Verification items for the finished model (mm, model axes). Face numbers are marked on the shaded views. A direction names the side the tool comes from. Round coordinates to 2 decimals unless told otherwise and drop trailing zeros. Write each loop counter-clockwise with the first axis right and the second up, starting at its lowest first coordinate (ties: lowest second). Pieces come first, ordered by that corner, then holes. Notation, with made-up numbers: M 3.5,49 L 55.5,49 A14 ccw 55.5,58 Z; hole C 63,26 d9. An arc over 180 degrees is marked long. One line per question, with ' | ' between items.
from build123d import *

# Parameters (mm, degrees)
F0_R     = 12.5
F0_R_2   = 18
F0_R_3   = 16
F0_R_4   = 8.5
F0_R_5   = 3.5
F1_DEPTH = 20
F2_DEPTH = 2
F3_R     = 1.5
F4_SIZE  = 1
F5_SIZE  = 1


# Not quite as in the source:
# - a feature names something its author has since deleted; it is built from what else it names


with BuildPart() as f1:
    # F0 (on Top) → F1 (new body)
    with BuildSketch(Plane.XY):
        with BuildLine():
            Line((82.5, 50), (-82.5, 50))
            ThreePointArc((-82.5, 50), (-86.0355339059, 48.5355339059), (-87.5, 45))
            Line((-87.5, 45), (-87.5, -45))
            ThreePointArc((-87.5, -45), (-86.0355339059, -48.5355339059), (-82.5, -50))
            Line((-82.5, -50), (82.5, -50))
            ThreePointArc((82.5, -50), (86.0355339059, -48.5355339059), (87.5, -45))
            Line((87.5, -45), (87.5, 45))
            ThreePointArc((87.5, 45), (86.0355339059, 48.5355339059), (82.5, 50))
        make_face()
        with Locations((-70, -34.5)):
            Circle(F0_R, mode=Mode.SUBTRACT)
        with BuildLine():
            ThreePointArc((-32.5, -34.5), (-45, -47), (-57.5, -34.5))
            ThreePointArc((-57.5, -34.5), (-45, -22), (-32.5, -34.5))
        make_face(mode=Mode.SUBTRACT)
        with BuildLine():
            ThreePointArc((-7.5, -34.5), (-20, -47), (-32.5, -34.5))
            ThreePointArc((-32.5, -34.5), (-20, -22), (-7.5, -34.5))
        make_face(mode=Mode.SUBTRACT)
        with Locations((-60, -3.5)):
            Circle(F0_R_2, mode=Mode.SUBTRACT)
        with Locations((-20, -3.5)):
            Circle(F0_R_2, mode=Mode.SUBTRACT)
        with BuildLine():
            ThreePointArc((17.5, -34.5), (5, -47), (-7.5, -34.5))
            ThreePointArc((-7.5, -34.5), (5, -22), (17.5, -34.5))
        make_face(mode=Mode.SUBTRACT)
        with BuildLine():
            ThreePointArc((20.5, -30.5), (22.5502525317, -25.5502525317), (27.5, -23.5))
            Line((27.5, -23.5), (77.5, -23.5))
            ThreePointArc((77.5, -23.5), (82.4497474683, -25.5502525317), (84.5, -30.5))
            Line((84.5, -30.5), (84.5, -38.5))
            ThreePointArc((84.5, -38.5), (82.4497474683, -43.4497474683), (77.5, -45.5))
            Line((77.5, -45.5), (27.5, -45.5))
            ThreePointArc((27.5, -45.5), (22.5502525317, -43.4497474683), (20.5, -38.5))
            Line((20.5, -38.5), (20.5, -30.5))
        make_face(mode=Mode.SUBTRACT)
        with Locations((20, -3.5)):
            Circle(F0_R_2, mode=Mode.SUBTRACT)
        with Locations((60, -3.5)):
            Circle(F0_R_2, mode=Mode.SUBTRACT)
        with BuildLine():
            ThreePointArc((82, 23), (79.9497474683, 18.0502525317), (75, 16))
            Line((75, 16), (-75, 16))
            ThreePointArc((-75, 16), (-79.9497474683, 18.0502525317), (-82, 23))
            Line((-82, 23), (-82, 40))
            ThreePointArc((-82, 40), (-79.9497474683, 44.9497474683), (-75, 47))
            Line((-75, 47), (75, 47))
            ThreePointArc((75, 47), (79.9497474683, 44.9497474683), (82, 40))
            Line((82, 40), (82, 23))
        make_face(mode=Mode.SUBTRACT)
        with BuildLine():
            Line((-75, 16), (75, 16))
            ThreePointArc((75, 16), (79.9497474683, 18.0502525317), (82, 23))
            Line((82, 23), (82, 40))
            ThreePointArc((82, 40), (79.9497474683, 44.9497474683), (75, 47))
            Line((75, 47), (-75, 47))
            ThreePointArc((-75, 47), (-79.9497474683, 44.9497474683), (-82, 40))
            Line((-82, 40), (-82, 23))
            ThreePointArc((-82, 23), (-79.9497474683, 18.0502525317), (-75, 16))
        make_face()
        with BuildLine():
            ThreePointArc((80, 23), (78.5355339059, 19.4644660941), (75, 18))
            Line((75, 18), (-75, 18))
            ThreePointArc((-75, 18), (-78.5355339059, 19.4644660941), (-80, 23))
            Line((-80, 23), (-80, 40))
            ThreePointArc((-80, 40), (-78.5355339059, 43.5355339059), (-75, 45))
            Line((-75, 45), (75, 45))
            ThreePointArc((75, 45), (78.5355339059, 43.5355339059), (80, 40))
            Line((80, 40), (80, 23))
        make_face(mode=Mode.SUBTRACT)
        with Locations((60, -3.5)):
            Circle(F0_R_2)
        with Locations((60, -3.5)):
            Circle(F0_R_3, mode=Mode.SUBTRACT)
        with Locations((20, -3.5)):
            Circle(F0_R_2)
        with Locations((20, -3.5)):
            Circle(F0_R_3, mode=Mode.SUBTRACT)
        with Locations((-20, -3.5)):
            Circle(F0_R_2)
        with Locations((-20, -3.5)):
            Circle(F0_R_3, mode=Mode.SUBTRACT)
        with Locations((-60, -3.5)):
            Circle(F0_R_2)
        with Locations((-60, -3.5)):
            Circle(F0_R_3, mode=Mode.SUBTRACT)
        with Locations((-70, -34.5)):
            Circle(F0_R)
        with Locations((-70, -34.5)):
            Circle(F0_R_4, mode=Mode.SUBTRACT)
        with Locations((-70, -34.5)):
            Circle(F0_R_4)
        with Locations((-70, -34.5)):
            Circle(F0_R_5, mode=Mode.SUBTRACT)
        with BuildLine():
            ThreePointArc((-32.5, -34.5), (-45, -22), (-57.5, -34.5))
            ThreePointArc((-57.5, -34.5), (-45, -47), (-32.5, -34.5))
        make_face()
        with Locations((-45, -34.5)):
            Circle(F0_R_4, mode=Mode.SUBTRACT)
        with Locations((-45, -34.5)):
            Circle(F0_R_4)
        with Locations((-45, -34.5)):
            Circle(F0_R_5, mode=Mode.SUBTRACT)
        with BuildLine():
            ThreePointArc((-7.5, -34.5), (-20, -22), (-32.5, -34.5))
            ThreePointArc((-32.5, -34.5), (-20, -47), (-7.5, -34.5))
        make_face()
        with Locations((-20, -34.5)):
            Circle(F0_R_4, mode=Mode.SUBTRACT)
        with Locations((-20, -34.5)):
            Circle(F0_R_4)
        with Locations((-20, -34.5)):
            Circle(F0_R_5, mode=Mode.SUBTRACT)
        with BuildLine():
            ThreePointArc((17.5, -34.5), (5, -22), (-7.5, -34.5))
            ThreePointArc((-7.5, -34.5), (5, -47), (17.5, -34.5))
        make_face()
        with Locations((5, -34.5)):
            Circle(F0_R_4, mode=Mode.SUBTRACT)
        with Locations((5, -34.5)):
            Circle(F0_R_4)
        with Locations((5, -34.5)):
            Circle(F0_R_5, mode=Mode.SUBTRACT)
        with BuildLine():
            Line((77.5, -23.5), (27.5, -23.5))
            ThreePointArc((27.5, -23.5), (22.5502525317, -25.5502525317), (20.5, -30.5))
            Line((20.5, -30.5), (20.5, -38.5))
            ThreePointArc((20.5, -38.5), (22.5502525317, -43.4497474683), (27.5, -45.5))
            Line((27.5, -45.5), (77.5, -45.5))
            ThreePointArc((77.5, -45.5), (82.4497474683, -43.4497474683), (84.5, -38.5))
            Line((84.5, -38.5), (84.5, -30.5))
            ThreePointArc((84.5, -30.5), (82.4497474683, -25.5502525317), (77.5, -23.5))
        make_face()
        with BuildLine():
            Line((27.5, -25.5), (77.5, -25.5))
            ThreePointArc((77.5, -25.5), (81.0355339059, -26.9644660941), (82.5, -30.5))
            Line((82.5, -30.5), (82.5, -38.5))
            ThreePointArc((82.5, -38.5), (81.0355339059, -42.0355339059), (77.5, -43.5))
            Line((77.5, -43.5), (27.5, -43.5))
            ThreePointArc((27.5, -43.5), (23.9644660941, -42.0355339059), (22.5, -38.5))
            Line((22.5, -38.5), (22.5, -30.5))
            ThreePointArc((22.5, -30.5), (23.9644660941, -26.9644660941), (27.5, -25.5))
        make_face(mode=Mode.SUBTRACT)
    extrude(amount=F1_DEPTH)

    # F0 (on Top) → F2 (join)
    with BuildSketch(Plane.XY):
        with Locations((-60, -3.5)):
            Circle(F0_R_3)
        with Locations((-20, -3.5)):
            Circle(F0_R_3)
        with Locations((60, -3.5)):
            Circle(F0_R_3)
        with BuildLine():
            Line((-75, 18), (75, 18))
            ThreePointArc((75, 18), (78.5355339059, 19.4644660941), (80, 23))
            Line((80, 23), (80, 40))
            ThreePointArc((80, 40), (78.5355339059, 43.5355339059), (75, 45))
            Line((75, 45), (-75, 45))
            ThreePointArc((-75, 45), (-78.5355339059, 43.5355339059), (-80, 40))
            Line((-80, 40), (-80, 23))
            ThreePointArc((-80, 23), (-78.5355339059, 19.4644660941), (-75, 18))
        make_face()
        with BuildLine():
            ThreePointArc((82.5, -30.5), (81.0355339059, -26.9644660941), (77.5, -25.5))
            Line((77.5, -25.5), (27.5, -25.5))
            ThreePointArc((27.5, -25.5), (23.9644660941, -26.9644660941), (22.5, -30.5))
            Line((22.5, -30.5), (22.5, -38.5))
            ThreePointArc((22.5, -38.5), (23.9644660941, -42.0355339059), (27.5, -43.5))
            Line((27.5, -43.5), (77.5, -43.5))
            ThreePointArc((77.5, -43.5), (81.0355339059, -42.0355339059), (82.5, -38.5))
            Line((82.5, -38.5), (82.5, -30.5))
        make_face()
        with Locations((20, -3.5)):
            Circle(F0_R_3)
    extrude(amount=F2_DEPTH)

    # F3
    f3_edges = [f1.edges().sort_by_distance(p)[0] for p in [
        (0, -50, 20),
    ]]
    fillet(f3_edges, radius=F3_R)

    # F4
    f4_edges = [f1.edges().sort_by_distance(p)[0] for p in [
        (-76, -3.5, 20),
        (-36, -3.5, 20),
        (44, -3.5, 20),
        (-78.535534, 43.535534, 20),
        (-80, 31.5, 20),
        (22.5, -30.5, 11),
        (23.964466, -26.964466, 20),
        (4, -3.5, 20),
    ]]
    chamfer(f4_edges, length=F4_SIZE)

    # F5
    f5_edges = [f1.edges().sort_by_distance(p)[0] for p in [
        (-73.5, -34.5, 20),
        (-48.5, -34.5, 20),
        (-23.5, -34.5, 20),
        (1.5, -34.5, 20),
    ]]
    chamfer(f5_edges, length=F5_SIZE)


solid = f1.part
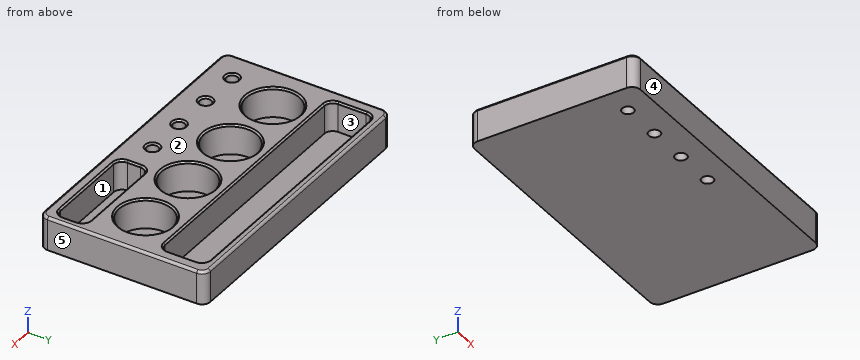
1. Tool access check on the marked faces 1 and 2. Record the directions out of +Z, -Z, +X, -X, +Y, -Y that give a thin tool (end or side, any length) a straight path to the whole face; none if there is none.
Results:
face 1: +Z | face 2: +Z, +X, -X, +Y, -Y
2. Section check D-D, the plane y = -34.5. Count the separate pieces of the cut face and the enclosed holes in it, then the cut area to 3 significant figures.
Results:
separate pieces: 5 | enclosed holes: 0 | area: 1,850 mm2
3. Section check A-A, the plane x = -20. Record the cut outline in (y, z).
Results:
outline: M -50,0 L -38,0 L -38,19 L -39,20 L -48.5,20 A1.5 ccw -50,18.5 Z; M -31,0 L 50,0 L 50,18.5 A1.5 ccw 48.5,20 L 46,20 L 45,19 L 45,2 L 18,2 L 18,19 L 17,20 L 13.5,20 L 12.5,19 L 12.5,2 L -19.5,2 L -19.5,19 L -20.5,20 L -30,20 L -31,19 Z
4. Section check C-C, the plane y = 34. Record the cut outline in (x, z).
Results:
outline: M -87.5,0 L 87.5,0 L 87.5,18.5 A1.5 ccw 86,20 L 81,20 L 80,19 L 80,2 L -80,2 L -80,19 L -81,20 L -86,20 A1.5 ccw -87.5,18.5 Z
5. Thickness scan on line 1 (Y direction, x = -20, z = 10.25); line 2 (Y direction, x = 60, z = 12.25); line 3 (Y direction, x = 20, z = 13.25). Record the ranges inside material, lowest first.
Results:
line 1: y = -50 to -38, -31 to -19.5, 12.5 to 18, 45 to 50 | line 2: y = -50 to -43.5, -25.5 to -19.5, 12.5 to 18, 45 to 50 | line 3: y = -50 to -19.5, 12.5 to 18, 45 to 50
6. Mould release check, pull along X, two halves, no side actions. Record for the marked faces 3, 4 and 5: pulls with the +X half, pulls with the -X half, needs draft (parallel to the pull), parting line crosses it, or undercut.
Results:
face 3: undercut | face 4: needs draft | face 5: pulls with the +X half
7. Go/stop test with flat-tipped pins: P1, Ø12, axis at x = 65.5, y = -39.5, coming from the -Z side; P2, Ø5.5, axis at x = 66.5, y = -38.5, coming from the +Z side; P3, Ø8, axis at x = -45, y = -34.5, coming from the +Z side. Record where each tip stops, or that it passes through.
Results:
P1: stops at z = 0 | P2: stops at z = 2 | P3: stops at z = 19.5
8. Section check B-B, the plane x = -60. Record the cut outline in (y, z).
Results:
outline: M -50,0 L 50,0 L 50,18.5 A1.5 ccw 48.5,20 L 46,20 L 45,19 L 45,2 L 18,2 L 18,19 L 17,20 L 13.5,20 L 12.5,19 L 12.5,2 L -19.5,2 L -19.5,19 L -20.5,20 L -48.5,20 A1.5 ccw -50,18.5 Z
